Here's how the part is built. I have some questions about the finished solid (model axes, mm). Face numbers are marked on the shaded views. A direction names the side the tool comes from. Coordinates: 2 decimals unless noted, no trailing zeros. Write each loop counter-clockwise with the first axis right and the second up, starting at its lowest first coordinate (ties: lowest second). Pieces come first, ordered by that corner, then holes.
Item 1: We'd pull the mould along X, two halves only. Please class the marked faces 1, 2 and 3: +X half, -X half, draft (parallel to the pull), parting line (faces both ways), or undercut.
Item 2: If I drill on line 1 (X direction, y = 10.5, z = 20.5); line 2 (Z direction, x = -0.5, y = 15.5); line 3 (X direction, y = 19.5, z = 14), over which ranges is the centre line in solid material (lowest first)?
Item 3: For the marked faces 4 and 5, which set-ups out of +Z, -Z, +X, -X, +Y, -Y let a thin tool reach every point of the face, with its end or its side?
Item 4: If we section it at B-B (y = 6.75): Please give me the cut outline in (x, z), then the cut area to 3 significant figures.
Item 5: If we section it at D-D (z = -38): Please give me the cut outline in (x, y), then the cut area to 3 significant figures.
Item 6: I'm going to push flat-ended pins straight in: pin 1 Ø1 at (x, z) = (-1.5, -24) entering from +Y; pin 2 Ø12 at (y, z) = (6.5, 33.5) entering from -X; pin 3 Ø8 at (y, z) = (11, 25.5) entering from +X. Where does each tip first touch, or does it pass through?
Item 7: If we section it at A-A (x = 0): Please give me the cut outline in (y, z).
Item 8: If we section it at C-C (z = 0): Please give me the cut outline in (x, y), then the cut area to 3 significant figures.
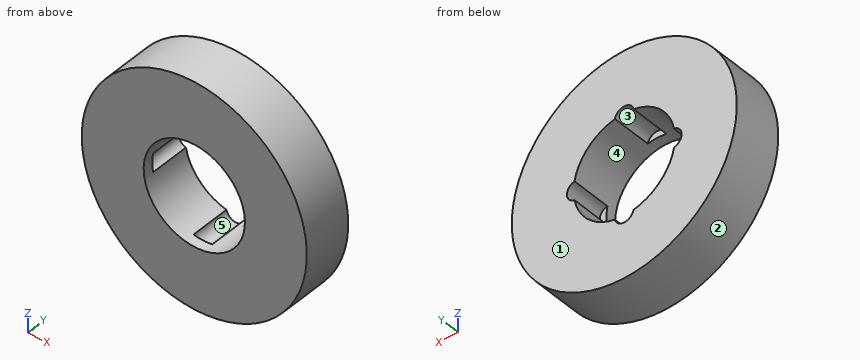
from build123d import *

# Parameters (mm, degrees)
SKETCH1_R           = 50
BOSS_EXTRUDE1_DEPTH = 22
SKETCH2_R           = 22.5
CUT_EXTRUDE1_DEPTH  = 75.054034326
SKETCH3_R           = 4.229056578
CUT_EXTRUDE2_DEPTH  = 17.438124
CIRPATTERN1_START   = 4.561875539
CIRPATTERN1_DEPTH   = 17.438124461


# Read off the part's stored shape, not the designer's step: CirPattern1
with BuildPart() as part:
    # Sketch1 → Boss-Extrude1 (new body)
    with BuildSketch(Plane(origin=(0, 0, 0), x_dir=(1, 0, 0), z_dir=(0, 1, 0))):
        with Locations(Location((0, 0, 0), (0, 0, 270))):
            Circle(SKETCH1_R)
    extrude(amount=BOSS_EXTRUDE1_DEPTH)

    # Sketch2 → Cut-Extrude1 (cut, through all)
    with BuildSketch(Plane(origin=(0, 0, 0), x_dir=(1, 0, 0), z_dir=(0, 1, 0))):
        with Locations(Location((0, 0, 0), (0, 0, 270))):
            Circle(SKETCH2_R)
    extrude(amount=CUT_EXTRUDE1_DEPTH, mode=Mode.SUBTRACT)

    # Sketch3 → Cut-Extrude2 (cut)
    with BuildSketch(Plane(origin=(0, 22, 0), x_dir=(1, 0, 0), z_dir=(0, 1, 0))):
        with Locations((-21.263269619, 0)):
            Circle(SKETCH3_R)
    extrude(amount=-CUT_EXTRUDE2_DEPTH, mode=Mode.SUBTRACT)

    # CirPattern1 outline → CirPattern1 (cut)
    with BuildSketch(Plane(origin=(0, 0, 0), x_dir=(1, 0, 0), z_dir=(0, 1, 0)).offset(CIRPATTERN1_START)):
        with BuildLine():
            ThreePointArc((-4.142315989, 22.115406807), (0, 22.5), (4.142315989, 22.115406807))
            ThreePointArc((4.142315989, 22.115406807), (0, 25.492326197), (-4.142315989, 22.115406807))
        make_face()
        with BuildLine():
            ThreePointArc((22.115406807, -4.142315989), (25.492326197, 0), (22.115406807, 4.142315989))
            ThreePointArc((22.115406807, 4.142315989), (22.5, 0), (22.115406807, -4.142315989))
        make_face()
        with BuildLine():
            ThreePointArc((4.142315989, -22.115406807), (0, -22.5), (-4.142315989, -22.115406807))
            ThreePointArc((-4.142315989, -22.115406807), (0, -25.492326197), (4.142315989, -22.115406807))
        make_face()
    extrude(amount=CIRPATTERN1_DEPTH, mode=Mode.SUBTRACT)


solid = part.part
Answer list:
1. face 1: draft
1. face 2: parting line
1. face 3: undercut
2. line 1: x = -45.6 to -9.27, 9.27 to 45.6
2. line 2: z = -50 to -25.46, 25.46 to 50
2. line 3: x = -48 to -17.61, 17.61 to 48
3. face 4: +Y, -Y
3. face 5: +Y
4. outline: circle Ø100 at (0, 0); hole (-22.12, -4.14) arc R22.5 ccw to (-4.14, -22.12) arc R4.23 ccw to (4.14, -22.12) arc R22.5 ccw to (22.12, -4.14) arc R4.23 ccw to (22.12, 4.14) arc R22.5 ccw to (4.14, 22.12) arc R4.23 ccw to (-4.14, 22.12) arc R22.5 ccw to (-22.12, 4.14) arc R4.23 ccw to start
4. area: 6,190 mm2
5. outline: (-32.5, 0) - (32.5, 0) - (32.5, 22) - (-32.5, 22) - close
5. area: 1,430 mm2
6. pin 1: stops at y = 4.56
6. pin 2: stops at x = -41.76
6. pin 3: stops at x = 45.14
7. outline: (0, -50) - (22, -50) - (22, -25.49) - (4.56, -25.49) - (4.56, -22.5) - (0, -22.5) - close; (0, 22.5) - (4.56, 22.5) - (4.56, 25.49) - (22, 25.49) - (22, 50) - (0, 50) - close
8. outline: (-50, 0) - (-22.5, 0) - (-22.5, 4.56) - (-25.49, 4.56) - (-25.49, 22) - (-50, 22) - close; (22.5, 0) - (50, 0) - (50, 22) - (25.49, 22) - (25.49, 4.56) - (22.5, 4.56) - close
8. area: 1,110 mm2
